from build123d import *

# Parameters (mm, degrees)
F0_R     = 7.62
F1_DEPTH = 1.27
F3_D     = 10.16
F4_W     = 3.81
F4_H     = 5.08
F5_DEPTH = 1.27


with BuildPart() as f1:
    # F0 (on Front) → F1 (new body, symmetric)
    with BuildSketch(Plane.XZ):
        Circle(F0_R)
    extrude(amount=F1_DEPTH, both=True)

    # F3 (through all)
    with Locations(Plane.XZ.offset(1.27)):
        with Locations((0, 0)):
            Hole(F3_D / 2)

    # F4 (on Front) → F5 (join, symmetric)
    with BuildSketch(Plane.XZ):
        with Locations((0.448802, -9.999485)):
            Rectangle(F4_W, F4_H)
        with BuildLine():
            Line((2.353802, -12.539485), (-1.456198, -12.539485))
            ThreePointArc((-1.456198, -12.539485), (11.08983, -11.3746), (16.51, 0))
            ThreePointArc((16.51, 0), (15.388414, 21.091942), (0, 35.56))
            ThreePointArc((0, 35.56), (-14.210098, 20.534478), (-16.665379, 0))
            Line((-16.665379, 0), (-12.7, 0))
            ThreePointArc((-12.7, 0), (-10.634561, 17.588824), (0, 31.75))
            ThreePointArc((0, 31.75), (12.493217, 18.332287), (12.7, 0))
            ThreePointArc((12.7, 0), (10.482185, -8.708117), (2.353802, -12.539485))
        make_face()
    extrude(amount=F5_DEPTH, both=True)


solid = f1.part
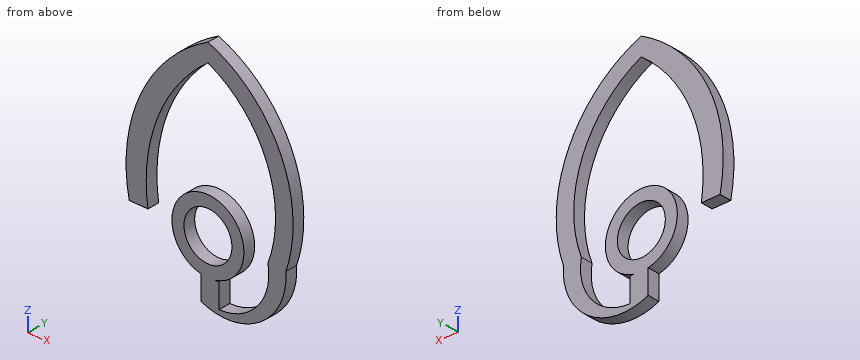
The listing builds one solid part. Answer for the finished solid, in the listing's coordinates (mm). Coordinates: 2 decimals unless noted, no trailing zeros. Loops run counter-clockwise (first coordinate to the right, second up) from the corner with the lowest first, then second, coordinate; pieces in that order, holes last. Notation, with made-up numbers: (33.5, -33) -> (90.5, -33) arc R23 cw to (90.5, 5) -> close; hole circle Ø8 at (-39, 67.25). An arc over 180 degrees is marked (long way). Write item = value, one per line. Start each with the question number.
1) A cutting plane is placed at A-A (y = -0.65). Give the vertices of the cut face in (x, z), then the cut area to 3 significant figures.
2) A cutting plane is placed at D-D (z = 14). Give the vertices of the cut face in (x, y), then the cut area to 3 significant figures.
3) A cutting plane is placed at B-B (z = 2). Give the vertices of the cut face in (x, y), then the cut area to 3 significant figures.
4) A cutting plane is placed at C-C (x = -3.5). Give the vertices of the cut face in (y, z).
5) Straight lines are drawn through the part: line 1 (Z direction, x = 6.5, y = -0.6); line 2 (X direction, y = -0.8, z = -4.5); line 3 (X direction, y = 0.4, z = 14). For each, find the intervals that lie inside material, in ascending order. Write a range as from..to.
6) Given pin 1 Ø0.8 at (x, y) = (-15, 0) entering from -Z; pin 2 Ø1.3 at (y, z) = (-0.5, -11) entering from -X; pin 3 Ø1 at (y, z) = (1, 10.5) entering from -X, each flat-ended and moving along its own axis, determine where each tip first touches the part or whether it passes through.
Responses:
q1.outline = (-16.67, 0) -> (-12.7, 0) arc R33.98 cw to (0, 31.75) arc R25.4 cw to (12.7, 0) arc R10.54 cw to (2.35, -12.54) -> (2.35, -7.46) -> (1.56, -7.46) arc R7.62 ccw (long way) to (-1.46, -7.48) -> (-1.46, -12.54) arc R12.75 ccw to (16.51, 0) arc R28.36 ccw to (0, 35.56) arc R32.95 ccw to start; hole circle Ø10.16 at (0, 0)
q1.area = 484 mm²
q2.outline = (-16.47, -1.27) -> (-11.84, -1.27) -> (-11.84, 1.27) -> (-16.47, 1.27) -> close; (13.79, -1.27) -> (17.61, -1.27) -> (17.61, 1.27) -> (13.79, 1.27) -> close
q2.area = 21.4 mm²
q3.outline = (-17.01, -1.27) -> (-12.94, -1.27) -> (-12.94, 1.27) -> (-17.01, 1.27) -> close; (-7.35, -1.27) -> (-4.67, -1.27) -> (-4.67, 1.27) -> (-7.35, 1.27) -> close; (4.67, -1.27) -> (7.35, -1.27) -> (7.35, 1.27) -> (4.67, 1.27) -> close; (13.36, -1.27) -> (17.11, -1.27) -> (17.11, 1.27) -> (13.36, 1.27) -> close
q3.area = 33.5 mm²
q4.outline = (-1.27, -6.77) -> (1.27, -6.77) -> (1.27, -3.68) -> (-1.27, -3.68) -> close; (-1.27, 3.68) -> (1.27, 3.68) -> (1.27, 6.77) -> (-1.27, 6.77) -> close; (-1.27, 28.6) -> (1.27, 28.6) -> (1.27, 33.38) -> (-1.27, 33.38) -> close
q5.line_1 = -13.38..-11.69, -3.98..3.98, 27.22..31.97
q5.line_2 = -6.15..-2.36, 2.36..6.15, 12.59..16.03
q5.line_3 = -16.47..-11.84, 13.79..17.61
q6.pin_1 = 0
q6.pin_2 = -1.46
q6.pin_3 = -17.14
